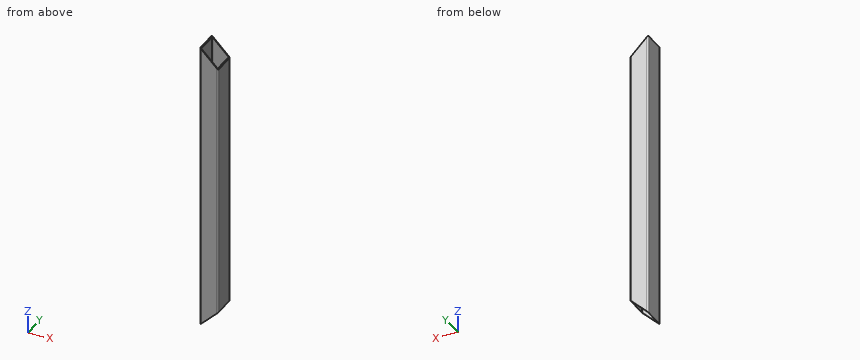
Autodesk Inventor part; units mm, degrees
ref_plane "Start plane" through (0, 0, 0) normal (0, 0, 1) x (1, 0, 0)
ref_plane "End plane" through (0, 0, 651) normal (0, 0, 1) x (1, 0, 0)
ref_plane "Work Plane4" through (-20, 0, 0) normal (0.7071, 0, -0.7071) x (-0.7071, 0, -0.7071)
ref_plane "Start plane" through (0, 0, 0) normal (0, 0, 1) x (1, 0, 0)
ref_plane "End plane" through (0, 0, 651) normal (0, 0, 1) x (1, 0, 0)
sketch "Sketch" plane through (0, 0, 0) normal (0, 0, 1) x (1, 0, 0)
  line L0 (-20, -22) -> (-20, 22)
  line L1 (-17, 25) -> (17, 25)
  line L2 (20, 22) -> (20, -22)
  line L3 (17, -25) -> (-17, -25)
  arc A0 (-20, -22) -> (-17, -25) centre (-17, -22) ccw
  arc A1 (-17, 25) -> (-20, 22) centre (-17, 22) ccw
  arc A2 (20, 22) -> (17, 25) centre (17, 22) ccw
  arc A3 (17, -25) -> (20, -22) centre (17, -22) ccw
  arc A4 (-17, 23) -> (-18, 22) centre (-17, 22) ccw
  line L4 (-17, 23) -> (17, 23)
  arc A5 (18, 22) -> (17, 23) centre (17, 22) ccw
  line L5 (18, 22) -> (18, -22)
  arc A6 (17, -23) -> (18, -22) centre (17, -22) ccw
  line L6 (17, -23) -> (-17, -23)
  arc A7 (-18, -22) -> (-17, -23) centre (-17, -22) ccw
  line L7 (-18, -22) -> (-18, 22)
  line L8 (0, 35.8698) -> (0, -35.8698) construction
  line L9 (-28.8698, 0) -> (28.8698, 0) construction
  dimension "d7" = 3
  dimension "d10" = 50
  dimension "d11" = 40
  dimension "d12" = 2
  dimension "d15" = 25
  dimension "d16" = 20
extrude "Body" add sketch "Sketch" along normal up to surface (651 mm away) from surface at 0
sketch "Sketch3" plane through (0, 0, 0) normal (0, 0, 1) x (1, 0, 0)
  line L0 (0, 0) -> (10, 0)
ref_plane "Work Plane3" through (0, 0, 0) normal (0, -1, 0) x (1, 0, 0)
sketch "Sketch4" plane through (0, 0, 0) normal (0, -1, 0) x (1, 0, 0)
  line L0 (-2, 0) -> (12, 0)
  line L1 (-2, 651) -> (12, 651)
  dimension "d18" = 651
ref_plane "Work Plane4" through (-20, 0, 0) normal (0.7071, 0, -0.7071) x (-0.7071, 0, -0.7071)
split "Split1" plane through (-20, 0, 0) removes the side toward (0.7071, 0, -0.7071)
ref_plane "Work Plane5" through (-20, 0, 651) normal (0.7071, 0, 0.7071) x (0.7071, 0, -0.7071)
split "Split2" plane through (-20, 0, 651) removes the side toward (0.7071, 0, 0.7071)
equation "\"d7\" = G_IR"
equation "\"d10\" = G_H"
equation "\"d11\" = G_W"
equation "\"d12\" = G_T"
equation "\"d15\" = 0.5 * d10"
equation "\"d16\" = 0.5 * d11"
equation "\"d3\" = G_L"
equation "\"G_W\" = 40"
equation "\"G_H\" = 50"
equation "\"G_T\" = 2"
equation "\"G_IR\" = 3"
equation "\"G_L\" = d18"
equation "\"G_OFFSET_START\" = 0"
equation "\"G_OFFSET_END\" = 0"
equation "\"d14\" = G_OFFSET_END + B_L"
equation "\"B_L\" = 651"
properties part number "UNI EN 10305-5 - 50 x 40 x 2  - 651" material "Steel, Mild"
The listing builds one solid part. Answer for the finished solid, in the listing's coordinates (mm). Give positions to 0.01 mm unless a question says otherwise; leave off trailing zeros. Loops run counter-clockwise (first coordinate to the right, second up) from the corner with the lowest first, then second, coordinate; pieces in that order, holes last. Notation, with made-up numbers: M -33,-35 L 12,-35 A23 ccw 12,-24 Z; hole C 59.25,-31 d4. An arc over 180 degrees is marked long. One line per item, written item: value.
Q1. Find the intervals of material crossed by line 1 (X direction, y = -14, z = 509); line 2 (Y direction, x = -0.5, z = 152.5); line 3 (Z direction, x = 13.5, y = 23.5), in increasing order. Write a range as from..to.
Working result:
line 1: x = -20..-18, 18..20
line 2: y = -25..-23, 23..25
line 3: z = 33.5..617.5
Q2. A cutting plane is placed at A-A on x = 11.5. Determine the outline of the cut face in (y, z), then the cut area to 3 significant figures.
Working result:
outline: M -25,31.5 L -23,31.5 L -23,619.5 L -25,619.5 Z; M 23,31.5 L 25,31.5 L 25,619.5 L 23,619.5 Z
area: 2,350 mm^2
Q3. A cutting plane is placed at B-B on z = 283. Determine the outline of the cut face in (x, y), then the cut area to 3 significant figures.
Working result:
outline: M -20,-22 A3 ccw -17,-25 L 17,-25 A3 ccw 20,-22 L 20,22 A3 ccw 17,25 L -17,25 A3 ccw -20,22 Z; hole M -18,-22 A1 ccw -17,-23 L 17,-23 A1 ccw 18,-22 L 18,22 A1 ccw 17,23 L -17,23 A1 ccw -18,22 Z
area: 337 mm^2
Q4. A cutting plane is placed at C-C on y = 8. Determine the outline of the cut face in (x, z), then the cut area to 3 significant figures.
Working result:
outline: M -20,0 L -18,2 L -18,649 L -20,651 Z; M 18,38 L 20,40 L 20,611 L 18,613 Z
area: 2,440 mm^2
